Read the model definition and answer for the solid it produces. Units are mm, in the model's axes. A direction names the side the tool comes from. Round coordinates to 2 decimals unless told otherwise and drop trailing zeros. Write each loop counter-clockwise with the first axis right and the second up, starting at its lowest first coordinate (ties: lowest second). Pieces come first, ordered by that corner, then holes. Notation, with made-up numbers: (-36, 59) - (15, 59) arc R27 cw to (15, 82) - close; hole circle Ø10 at (61, 29.5). An arc over 180 degrees is marked (long way). One line per item, written item: value. Start each with the question number.
(1) A cutting plane is placed at A-A, the plane z = 0. Determine the outline of the cut face in (x, y) (3 decimals), plus the area to 3 significant figures.
(2) Flat-ended cylindrical pins translate along their axes: pin 1 Ø1.5 at (y, z) = (27.5, 4) entering from -X; pin 2 Ø12 at (x, z) = (-8, 6.5) entering from -Y; pin 3 Ø12 at (y, z) = (62.5, 0.5) entering from +X; pin 4 Ø10 at (x, y) = (6, 70.5) entering from +Z. Find the tip coordinate at first contact, or state that the pin passes through.
(3) For faces 1 (the face through (-2, 76.895, 0)), 2 (the face through (-0.54, 82.16, 2.44)), 3 (the face through (0, 84.495, 0)), determine the directions among +Z, -Z, +X, -X, +Y, -Y from which every point of the face is accessible in a straight line to the end or side of a thin tool.
(4) A cutting plane is placed at C-C, the plane y = 74. Determine the outline of the cut face in (x, z).
(5) Find the intervals of material crossed by L1, parallel to Y at x = -1.5, z = -11; L2, parallel to Y at x = 4, z = -8; L3, parallel to X at y = 50.5, z = 2, in increasing order.
(6) A cutting plane is placed at B-B, the plane x = 0. Determine the outline of the cut face in (y, z) (3 decimals).
(7) The mould has two halves that part along Y. Classify faces 4 (the face through (2, 79.895, 0)), 5 (the face through (-1.48, 4.98, 6.65)), 6 (the face through (-2.93, 1.5, 13.18)): +Y half, -Y half, draft (parallel to the pull), parting line (faces both ways), or undercut.
from build123d import *


with BuildPart() as part:
    # Sketch1 → Revolve1 (revolve)
    with BuildSketch(Plane.XY):
        with BuildLine():
            Line((0, 0), (0, 84.495))
            Line((0, 84.495), (2.5, 84.495))
            Line((2.5, 84.495), (2.5, 79.895))
            Line((2.5, 79.895), (1.5, 79.895))
            Line((1.5, 79.895), (1.5, 76.895))
            Line((1.5, 76.895), (2.5, 76.895))
            Line((2.5, 76.895), (2.5, 10.749955013))
            ThreePointArc((2.5, 10.749955013), (3.585087734, 7.308496395), (6.44787914, 5.111799289))
            Line((6.44787914, 5.111799289), (12.25, 3))
            Line((12.25, 3), (13.5, 1.75))
            Line((13.5, 1.75), (13.5, 1.25))
            ThreePointArc((13.5, 1.25), (6.778873431, 0.31316694), (0, 0))
        make_face()
    revolve(axis=Axis((0, 0, 0), (0, 1, 0)))


solid = part.part
Here are the results:
1. outline: (-13.5, 1.25) arc R73.525 ccw to (13.5, 1.25) - (13.5, 1.75) - (12.25, 3) - (6.448, 5.112) arc R6 cw to (2.5, 10.75) - (2.5, 76.895) - (1.5, 76.895) - (1.5, 79.895) - (2.5, 79.895) - (2.5, 84.495) - (-2.5, 84.495) - (-2.5, 79.895) - (-1.5, 79.895) - (-1.5, 76.895) - (-2.5, 76.895) - (-2.5, 10.75) arc R6 cw to (-6.448, 5.112) - (-12.25, 3) - (-13.5, 1.75) - close
1. area: 511 mm²
2. pin 1: through
2. pin 2: y = 0.13
2. pin 3: x = 2.5
2. pin 4: z = 2.29
3. face 1: none
3. face 2: +Y
3. face 3: +Z, -Z, +X, -X, +Y
4. outline: circle Ø5 at (0, 0)
5. L1: 0.84 to 3.42
5. L2: 0.55 to 4.2
5. L3: -1.5 to 1.5
6. outline: (1.25, -13.5) - (1.75, -13.5) - (3, -12.25) - (5.112, -6.448) arc R6 cw to (10.75, -2.5) - (76.895, -2.5) - (76.895, -1.5) - (79.895, -1.5) - (79.895, -2.5) - (84.495, -2.5) - (84.495, 2.5) - (79.895, 2.5) - (79.895, 1.5) - (76.895, 1.5) - (76.895, 2.5) - (10.75, 2.5) arc R6 cw to (5.112, 6.448) - (3, 12.25) - (1.75, 13.5) - (1.25, 13.5) arc R73.525 ccw to start
7. face 4: undercut
7. face 5: +Y half
7. face 6: draft
